```python
from build123d import *

# Parameters (mm, degrees)
SKETCH_2_W           = 40
SKETCH_2_H           = 25
EXTRUDE_1_DEPTH      = 5
SKETCH_3_R           = 1.5
CUT_EXTRUDE_1_DEPTH  = 25.109126902
SKETCH_4_R           = 5
CUT_EXTRUDE_2_DEPTH  = 25.109126902
EXTRUDE_2_DEPTH      = 12.5
EXTRUDE_2_DEPTH_BACK = 12.5
SKETCH_7_R           = 5
SKETCH_7_R_2         = 1.5
CUT_EXTRUDE_3_DEPTH  = 43.405777908
FILLET_1_R           = 5
FILLET_2_R           = 1


with BuildPart() as part:
    # 草图2 → 凸台-拉伸1 (new body)
    with BuildSketch(Plane.XY):
        Rectangle(SKETCH_2_W, SKETCH_2_H)
    extrude(amount=EXTRUDE_1_DEPTH)

    # 草图3 → 切除-拉伸1 (cut, through all)
    with BuildSketch(Plane.XY.offset(5)):
        with Locations((-15, 8)):
            Circle(SKETCH_3_R)
        with Locations((0, 8)):
            Circle(SKETCH_3_R)
        with Locations(Location((15, 8, 0), (0, 0, 180))):
            Circle(SKETCH_3_R)
        with Locations((15, -8)):
            Circle(SKETCH_3_R)
        with Locations(Location((0, -8, 0), (0, 0, 180))):
            Circle(SKETCH_3_R)
        with Locations(Location((-15, -8, 0), (0, 0, 180))):
            Circle(SKETCH_3_R)
    extrude(amount=-CUT_EXTRUDE_1_DEPTH, mode=Mode.SUBTRACT)

    # 草图4 → 切除-拉伸2 (cut, through all)
    with BuildSketch(Plane.XY.offset(5)):
        with Locations((-7.5, 0)):
            Circle(SKETCH_4_R)
        with Locations(Location((7.5, 0, 0), (0, 0, 180))):
            Circle(SKETCH_4_R)
    extrude(amount=-CUT_EXTRUDE_2_DEPTH, mode=Mode.SUBTRACT)

    # 草图6 → 凸台-拉伸2 (add, two sides: drawn at the far end of the back side and taken through both)
    with BuildSketch(Plane(origin=(0, 0, 0), x_dir=(1, 0, 0), z_dir=(0, 1, 0)).offset(-EXTRUDE_2_DEPTH_BACK)):
        with BuildLine():
            Line((-20, -5), (-22, -5))
            ThreePointArc((-22, -5), (-30.488746876, -6.045012495), (-38.470588235, -9.117647059))
            ThreePointArc((-38.470588235, -9.117647059), (-38.9701425, -10.242535625), (-38, -11))
            Line((-38, -11), (20, -11))
            Line((20, -11), (20, -5))
            Line((20, -5), (-20, -5))
        make_face()
    extrude(amount=EXTRUDE_2_DEPTH + EXTRUDE_2_DEPTH_BACK)

    # 草图7 → 切除-拉伸3 (cut, through all)
    with BuildSketch(Plane.XY.offset(11)):
        with Locations((7.5, 0)):
            Circle(SKETCH_7_R)
        with Locations((-15, -8)):
            Circle(SKETCH_7_R_2)
        with Locations((-7.5, 0)):
            Circle(SKETCH_7_R)
        with Locations((0, -8)):
            Circle(SKETCH_7_R_2)
        with Locations((15, -8)):
            Circle(SKETCH_7_R_2)
        with Locations((0, 8)):
            Circle(SKETCH_7_R_2)
        with Locations((-15, 8)):
            Circle(SKETCH_7_R_2)
        with Locations((15, 8)):
            Circle(SKETCH_7_R_2)
    extrude(amount=-CUT_EXTRUDE_3_DEPTH, mode=Mode.SUBTRACT)

    # 圆角1
    fillet_1_edges = [part.edges().sort_by_distance(p)[0] for p in [
        (20, -12.5, 5.5),
        (-20, -12.5, 2.5),
        (-20, 12.5, 2.5),
        (20, 12.5, 5.5),
    ]]
    fillet(fillet_1_edges, radius=FILLET_1_R)

    # 圆角2
    # the kernel refuses this fillet: 1 mm, written as the material it adds along each edge
    with BuildSketch(Plane(origin=(-20, 7.5, 5), x_dir=(0, 0, -1), z_dir=(0, -1, 0))) as fillet_2_piece_1:
        with BuildLine():
            CenterArc((FILLET_2_R, -FILLET_2_R), FILLET_2_R, 90, 90)
            Line((0, -FILLET_2_R), (0, 0))
            Line((0, 0), (FILLET_2_R, 0))
        make_face()
    extrude(amount=15)
    with BuildSketch(Plane(origin=(-15, -7.5, 5), x_dir=(0.7515057138603054, -0.6597265812708418, 0), z_dir=(0.6597265812708418, 0.7515057138603054, 0))) as fillet_2_piece_2_section:
        with BuildLine():
            CenterArc((5 + FILLET_2_R, FILLET_2_R), FILLET_2_R, 180, 90)
            Line((5, FILLET_2_R), (5, 0))
            Line((5, 0), (5 + FILLET_2_R, 0))
        make_face()
    fillet_2_piece_2 = revolve(axis=Axis((-15, -7.5, 5), (0, 0, -1)), revolution_arc=138.720976341, mode=Mode.PRIVATE)
    fillet_2_piece_2 = split(fillet_2_piece_2, bisect_by=Plane(origin=(-15, -12.5, 5), z_dir=(0, 1, 0)), keep=Keep.TOP, mode=Mode.PRIVATE)
    add(fillet_2_piece_2)
    with BuildSketch(Plane(origin=(-15, 7.5, 5), x_dir=(0.7515057138603056, 0.6597265812708417, 0), z_dir=(0.6597265812708417, -0.7515057138603056, 0))) as fillet_2_piece_3_section:
        with BuildLine():
            CenterArc((5 + FILLET_2_R, -FILLET_2_R), FILLET_2_R, 90, 90)
            Line((5 + FILLET_2_R, 0), (5, 0))
            Line((5, 0), (5, -FILLET_2_R))
        make_face()
    fillet_2_piece_3 = revolve(axis=Axis((-15, 7.5, 5), (0, 0, 1)), revolution_arc=138.720976341, mode=Mode.PRIVATE)
    fillet_2_piece_3 = split(fillet_2_piece_3, bisect_by=Plane(origin=(-15, 12.5, 5), z_dir=(0, -1, 0)), keep=Keep.TOP, mode=Mode.PRIVATE)
    add(fillet_2_piece_3)


solid = part.part
```
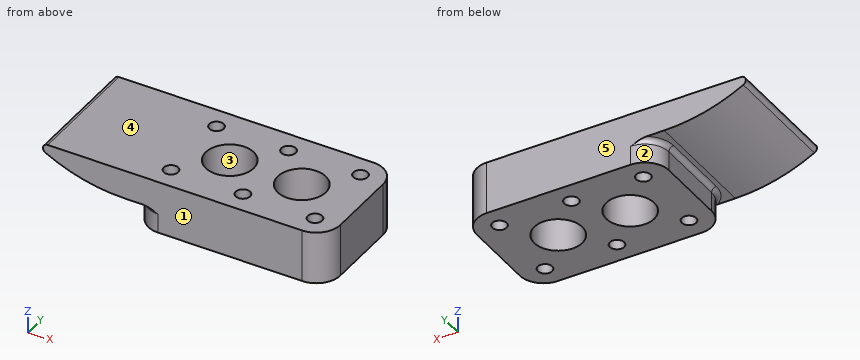
CAD build for the part. Positions are in the model's coordinates, mm. Face numbers are marked on the shaded views. A direction names the side the tool comes from. Coordinates: 2 decimals unless noted, no trailing zeros. Order: outer loops, then holes, each group sorted by start corner. A loop starts at its lowest first (then second) coordinate and runs counter-clockwise, first axis right, second up. Notation, with made-up numbers: (32, -2.5) -> (50, -2.5) arc R22 cw to (50, 10.5) -> close; hole circle Ø11 at (-20, -32). An arc over 180 degrees is marked (long way). Use one line per item in the form item = value. Start each with the question number.
1) Drill centre lines: L1, parallel to Y at x = 15, z = 3.25; L2, parallel to X at y = -1.25, z = 10.25; L3, parallel to Y at x = 7.5, z = 6.75. Where is each one in solid material? Low to high. Write a range as [from, to].
2) Band-saw the part on B-B on z = 2.5. State how many separate pieces and enclosed holes the cut face has, then the cut area to 3 significant figures.
3) Band-saw the part on D-D on y = 3.5. Give the cut face in (x, z).
4) Band-saw the part on C-C on x = 0. Give the cut face in (y, z).
5) Tool access for the marked faces 1 and 2: list every direction of +Z, -Z, +X, -X, +Y, -Y with a clear straight run to the whole face (end or side of a thin tool).
6) Band-saw the part on A-A on x = 7.5. Give the cut face in (y, z), then the cut area to 3 significant figures.
7) Pull direction Y, two halves, no side cores. Call the marked faces 3, 4 and 5: +Y half, -Y half, draft (parallel to the pull), parting line (faces both ways), or undercut.
8) Drop flat-ended pins along their axis: pin 1 (3 mm diameter, centred on y = -1, z = 3, fed in from -X); pin 2 (4 mm diameter, centred on y = -8, z = 6.5, fed in from -X); pin 3 (4 mm diameter, centred on x = -21.5, z = 2, fed in from -Y). Give the stop position or say it passes through.
Entries:
q1.L1 = [-12.5, -9.5], [-6.5, 6.5], [9.5, 12.5]
q1.L2 = [-38.97, -12.34], [-2.66, 2.66], [12.34, 20]
q1.L3 = [-12.5, -5], [5, 12.5]
q2.separate_pieces = 1
q2.enclosed_holes = 8
q2.area = 779 mm2
q3.outline = (-38.47, 9.12) arc R35 ccw to (-22, 5) -> (-21, 5) arc R1 cw to (-20, 4) -> (-20, 0) -> (-11.07, 0) -> (-11.07, 11) -> (-38, 11) arc R1 ccw to start; (-3.93, 0) -> (3.93, 0) -> (3.93, 11) -> (-3.93, 11) -> close; (11.07, 0) -> (20, 0) -> (20, 11) -> (11.07, 11) -> close
q4.outline = (-12.5, 0) -> (-9.5, 0) -> (-9.5, 11) -> (-12.5, 11) -> close; (-6.5, 0) -> (6.5, 0) -> (6.5, 11) -> (-6.5, 11) -> close; (9.5, 0) -> (12.5, 0) -> (12.5, 11) -> (9.5, 11) -> close
q5.face_1 = +Z, -Z, +X, -X, -Y
q5.face_2 = -Z, -X, +Y
q6.outline = (-12.5, 0) -> (-5, 0) -> (-5, 11) -> (-12.5, 11) -> close; (5, 0) -> (12.5, 0) -> (12.5, 11) -> (5, 11) -> close
q6.area = 165 mm2
q7.face_3 = undercut
q7.face_4 = draft
q7.face_5 = +Y half
q8.pin_1 = -20.13
q8.pin_2 = -37.26
q8.pin_3 = -9.68
